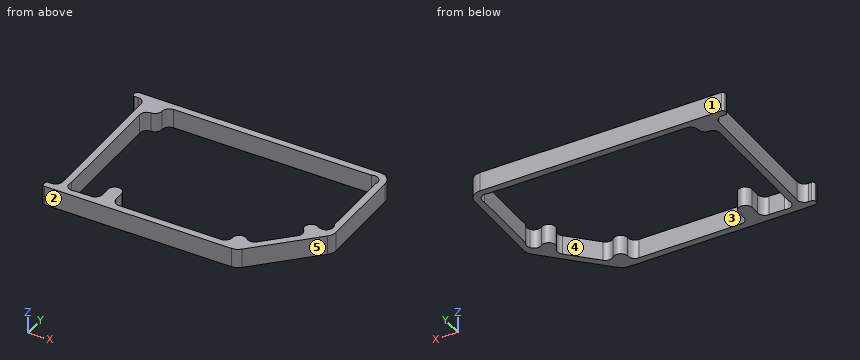
from build123d import *

# Parameters (mm, degrees)
BOSS_EXTRUDE1_DEPTH = 8.5


with BuildPart() as part:
    # Sketch1 → Boss-Extrude1 (new body)
    with BuildSketch(Plane.XY):
        with BuildLine():
            Line((-8.87, -1.3), (-8.87, -2.3))
            ThreePointArc((-8.87, -2.3), (-8.577106781, -3.007106781), (-7.87, -3.3))
            Line((-7.87, -3.3), (74.171572667, -3.3))
            ThreePointArc((74.171572667, -3.3), (76.199795144, -2.896561433), (77.919239112, -1.747665644))
            Line((77.919239112, -1.747665644), (101.747665711, 22.080760955))
            ThreePointArc((101.747665711, 22.080760955), (102.896561433, 23.800204856), (103.3, 25.828427238))
            Line((103.3, 25.828427238), (103.3, 63))
            ThreePointArc((103.3, 63), (101.74766594, 66.74766594), (98, 68.3))
            Line((98, 68.3), (-7.87, 68.3))
            ThreePointArc((-7.87, 68.3), (-8.577106781, 68.007106781), (-8.87, 67.3))
            Line((-8.87, 67.3), (-8.87, 66.3))
            ThreePointArc((-8.87, 66.3), (-8.577106781, 65.592893219), (-7.87, 65.3))
            Line((-7.87, 65.3), (-6.475, 65.3))
            ThreePointArc((-6.475, 65.3), (-4.22993597, 64.37006403), (-3.3, 62.125))
            Line((-3.3, 62.125), (-3.3, 2.875))
            ThreePointArc((-3.3, 2.875), (-4.22993597, 0.62993597), (-6.475, -0.3))
            Line((-6.475, -0.3), (-7.87, -0.3))
            ThreePointArc((-7.87, -0.3), (-8.577106781, -0.592893219), (-8.87, -1.3))
        make_face()
        with BuildLine():
            Line((100.2, 29.856417462), (100.2, 60.994582891))
            ThreePointArc((100.2, 60.994582891), (99.555634919, 64.555634919), (95.994582891, 65.2))
            Line((95.994582891, 65.2), (9.175, 65.2))
            ThreePointArc((9.175, 65.2), (6.92993597, 64.27006403), (6, 62.025))
            Line((6, 62.025), (6, 62))
            ThreePointArc((6, 62), (5.121320344, 59.878679656), (3, 59))
            Line((3, 59), (2.975, 59))
            ThreePointArc((2.975, 59), (0.72993597, 58.07006403), (-0.2, 55.825))
            Line((-0.2, 55.825), (-0.2, 4.005417109))
            ThreePointArc((-0.2, 4.005417109), (0.444365081, 0.444365081), (4.005417109, -0.2))
            Line((4.005417109, -0.2), (10.825, -0.2))
            ThreePointArc((10.825, -0.2), (13.07006403, 0.72993597), (14, 2.975))
            Line((14, 2.975), (14, 7))
            ThreePointArc((14, 7), (17, 10), (20, 7))
            Line((20, 7), (20, 2.975))
            ThreePointArc((20, 2.975), (20.92993597, 0.72993597), (23.175, -0.2))
            Line((23.175, -0.2), (67.825, -0.2))
            ThreePointArc((67.825, -0.2), (70.07006403, 0.72993597), (71, 2.975))
            Line((71, 2.975), (71, 3))
            ThreePointArc((71, 3), (72.819133757, 5.757817056), (76.070369945, 5.171075377))
            ThreePointArc((76.070369945, 5.171075377), (78.299195815, 4.294020465), (80.5065755, 5.223732787))
            Line((80.5065755, 5.223732787), (91.776267213, 16.4934245))
            ThreePointArc((91.776267213, 16.4934245), (92.705979535, 18.700804185), (91.828924623, 20.929630055))
            ThreePointArc((91.828924623, 20.929630055), (91.741164129, 24.974249353), (95.761133603, 25.428663919))
            ThreePointArc((95.761133603, 25.428663919), (98.192543935, 24.875137086), (100.273869597, 26.248538573))
            ThreePointArc((100.273869597, 26.248538573), (100.79933472, 28.063992887), (100.2, 29.856417462))
        make_face(mode=Mode.SUBTRACT)
    extrude(amount=BOSS_EXTRUDE1_DEPTH)


solid = part.part
Geometry: final body of the model. Coordinates: model frame, mm. Face numbers are marked on the shaded views. A direction names the side the tool comes from. Give positions to 0.01 mm unless a question says otherwise; leave off trailing zeros. Write each loop counter-clockwise with the first axis right and the second up, starting at its lowest first coordinate (ties: lowest second). Pieces come first, ordered by that corner, then holes.
(1) Mould query, pull axis Y, two halves, no side actions, for the marked faces 1, 2 and 3. Classes: released by +Y, released by -Y, zero draft, split by the parting line, or undercut.
(2) Access query for the marked faces 4 and 5. Directions: +Z, -Z, +X, -X, +Y, -Y. A direction counts if a zero-diameter tool reaches every point of the face in a straight line with its end or side. Return the directions, or none.
(3) First-contact query: P1, Ø4, axis at y = 35, z = 4.5, coming from the -X side; P2, Ø2, axis at y = 4, z = 4.5, coming from the +X side; P3, Ø5, axis at x = 90.5, z = 7, coming from the -Y side. Flat tips, straight axial feed; report the tip coordinate or a pass-through.
(4) Cut plane A-A, the plane x = 17. Return loops of the section in (y, z), then the cut area to 3 significant figures.
(5) Cut plane B-B, the plane y = 52. Return loops of the section in (x, z), then the cut area to 3 significant figures.
(6) Ray query, line 1 (Y direction, x = 43, z = 1); line 2 (X direction, y = 57, z = 5.5); line 3 (X direction, y = 1.5, z = 5.5). Return the intervals inside material, ascending.
Values follow:
1. face 1: released by +Y
1. face 2: released by -Y
1. face 3: undercut
2. face 4: +Z, -Z
2. face 5: +Z, -Z, +X, -Y
3. P1: stops at x = -3.3
3. P2: stops at x = 84.67
3. P3: stops at y = 8.33
4. outline: (-3.3, 0) - (10, 0) - (10, 8.5) - (-3.3, 8.5) - close; (65.2, 0) - (68.3, 0) - (68.3, 8.5) - (65.2, 8.5) - close
4. area: 139 mm2
5. outline: (-3.3, 0) - (-0.2, 0) - (-0.2, 8.5) - (-3.3, 8.5) - close; (100.2, 0) - (103.3, 0) - (103.3, 8.5) - (100.2, 8.5) - close
5. area: 52.7 mm2
6. line 1: y = -3.3 to -0.2, 65.2 to 68.3
6. line 2: x = -3.3 to 0.03, 100.2 to 103.3
6. line 3: x = -3.61 to -0.25, 13.64 to 20.36, 70.64 to 81.17
